Verification items for the finished model (mm, model axes). Face numbers are marked on the shaded views. Round coordinates to 2 decimals unless told otherwise and drop trailing zeros. One line per question, with ' | ' between items.
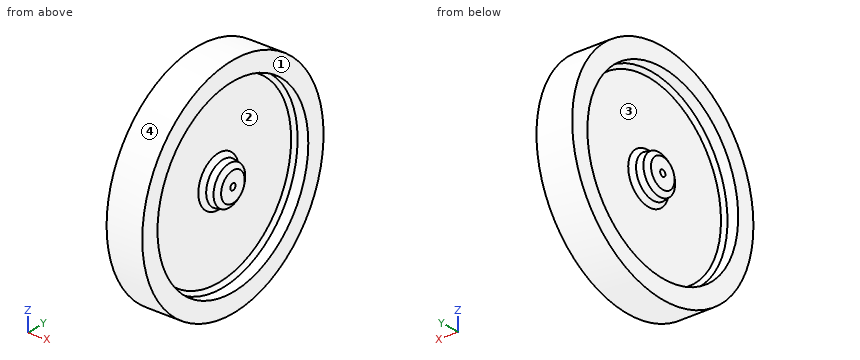
from build123d import *

# Parameters (mm, degrees)
SKETCH1_W           = 10
SKETCH1_H           = 31.25
SKETCH2_R           = 26
CUT_EXTRUDE1_DEPTH  = 4
SKETCH3_R           = 6
BOSS_EXTRUDE1_DEPTH = 4
BOSS_EXTRUDE1_TAPER = 10
CUT_EXTRUDE2_START  = -4
SKETCH4_R           = 26
CUT_EXTRUDE2_DEPTH  = 4
SKETCH5_R           = 6
BOSS_EXTRUDE2_DEPTH = 4
BOSS_EXTRUDE2_TAPER = 10
CHAMFER1_SIZE       = 1
CHAMFER1_SIZE_2     = 1.232803052
SKETCH6_R           = 0.9
CUT_EXTRUDE3_DEPTH  = 46.311422401


with BuildPart() as part:
    # Sketch1 → Revolve1 (revolve)
    with BuildSketch(Plane.XY):
        with Locations((0, -15.625)):
            Rectangle(SKETCH1_W, SKETCH1_H)
    revolve(axis=Axis((-5, 0, 0), (1, 0, 0)))

    # Sketch2 → Cut-Extrude1 (cut)
    with BuildSketch(Plane(origin=(5, 0, 0), x_dir=(0, 0, -1), z_dir=(1, 0, 0))):
        with Locations(Location((0, 0, 0), (0, 0, 90))):
            Circle(SKETCH2_R)
    extrude(amount=-CUT_EXTRUDE1_DEPTH, mode=Mode.SUBTRACT)

    # Sketch3 → Boss-Extrude1 (add)
    with BuildSketch(Plane(origin=(1, 0, 0), x_dir=(0, 0, -1), z_dir=(1, 0, 0))):
        Circle(SKETCH3_R)
    extrude(amount=BOSS_EXTRUDE1_DEPTH, taper=BOSS_EXTRUDE1_TAPER)

    # Sketch4 → Cut-Extrude2 (cut)
    with BuildSketch(Plane.ZY.offset(5).offset(CUT_EXTRUDE2_START)):
        with Locations(Location((0, 0, 0), (0, 0, 90))):
            Circle(SKETCH4_R)
    extrude(amount=CUT_EXTRUDE2_DEPTH, mode=Mode.SUBTRACT)

    # Sketch5 → Boss-Extrude2 (add)
    with BuildSketch(Plane.ZY.offset(1)):
        Circle(SKETCH5_R)
    extrude(amount=BOSS_EXTRUDE2_DEPTH, taper=BOSS_EXTRUDE2_TAPER)

    # Chamfer1
    # the kernel refuses this chamfer: 1.232803052, 1 mm, written as the material it adds along each edge
    with BuildSketch(Plane(origin=(1, 0, 0), x_dir=(0, 0, -1), z_dir=(0, -1, 0))) as chamfer1_piece_1:
        Polygon((6 + CHAMFER1_SIZE, 0), (6 - CHAMFER1_SIZE_2 * 0.173648177642, CHAMFER1_SIZE_2 * 0.98480775287), (6, 0), align=None)
    revolve(axis=Axis((1, 0, 0), (1, 0, 0)))
    with BuildSketch(Plane(origin=(-1, 0, 0), x_dir=(0, 1, 0), z_dir=(0, 0, 1))) as chamfer1_piece_2:
        Polygon((26, CHAMFER1_SIZE), (26 - CHAMFER1_SIZE, 0), (26, 0), align=None)
    revolve(axis=Axis((-1, 0, 0), (-1, 0, 0)))
    with BuildSketch(Plane(origin=(1, 0, 0), x_dir=(0, 1, 0), z_dir=(0, 0, -1))) as chamfer1_piece_3:
        Polygon((26, CHAMFER1_SIZE), (26 - CHAMFER1_SIZE, 0), (26, 0), align=None)
    revolve(axis=Axis((1, 0, 0), (1, 0, 0)))
    with BuildSketch(Plane(origin=(-1, 0, 0), x_dir=(0, 0, 1), z_dir=(0, -1, 0))) as chamfer1_piece_4:
        Polygon((6 + CHAMFER1_SIZE, 0), (6 - CHAMFER1_SIZE_2 * 0.173648177642, CHAMFER1_SIZE_2 * 0.98480775287), (6, 0), align=None)
    revolve(axis=Axis((-1, 0, 0), (-1, 0, 0)))
    # the kernel refuses this chamfer: 1.232803052, 1 mm, written as the material it takes off along each edge
    with BuildSketch(Plane(origin=(5, 0, 0), x_dir=(0, 0, -1), z_dir=(0, 1, 0))) as chamfer1_2_piece_1:
        Polygon((5.294692077 + CHAMFER1_SIZE * 0.173648177667, CHAMFER1_SIZE * 0.984807753012), (5.294692077 - CHAMFER1_SIZE_2, 0), (5.294692077, 0), align=None)
    revolve(axis=Axis((5, 0, 0), (-1, 0, 0)), mode=Mode.SUBTRACT)
    with BuildSketch(Plane(origin=(-5, 0, 0), x_dir=(0, 0, 1), z_dir=(0, 1, 0))) as chamfer1_2_piece_2:
        Polygon((5.294692077 + CHAMFER1_SIZE * 0.173648177667, CHAMFER1_SIZE * 0.984807753012), (5.294692077 - CHAMFER1_SIZE_2, 0), (5.294692077, 0), align=None)
    revolve(axis=Axis((-5, 0, 0), (1, 0, 0)), mode=Mode.SUBTRACT)

    # Sketch6 → Cut-Extrude3 (cut, through all)
    with BuildSketch(Plane.ZY.offset(5)):
        with Locations(Location((0, 0, 0), (0, 0, 270))):
            Circle(SKETCH6_R)
    extrude(amount=-CUT_EXTRUDE3_DEPTH, mode=Mode.SUBTRACT)


solid = part.part
1. Thickness scan on line 1 (Z direction, x = 3.5, y = 0); line 2 (X direction, y = 7.5, z = 0); line 3 (Y direction, x = 4.25, z = 1). Record the ranges inside material, lowest first.
Results:
line 1: z = -31.25 to -26, -5.56 to -0.9, 0.9 to 5.56, 26 to 31.25 | line 2: x = -1 to 1 | line 3: y = -31.23 to -25.98, -5.03 to 5.03, 25.98 to 31.23
2. Mould release check, pull along Z, two halves, no side actions. Record for the marked faces 1, 2, 3 and 4: pulls with the +Z half, pulls with the -Z half, needs draft (parallel to the pull), parting line crosses it, or undercut.
Results:
face 1: needs draft | face 2: undercut | face 3: undercut | face 4: parting line crosses it
3. Go/stop test with flat-tipped pins: P1, Ø1, axis at x = 2.5, y = -18.5, coming from the +Z side; P2, Ø12, axis at y = 9, z = -17, coming from the -X side; P3, Ø15, axis at y = -3.5, z = -10, coming from the -X side; P4, Ø12, axis at y = -14.5, z = -7, coming from the -X side. Record where each tip stops, or that it passes through.
Results:
P1: stops at z = 25.55 | P2: stops at x = -1.24 | P3: stops at x = -5 | P4: stops at x = -1
